For this review, use the dimensioned drawing (mm, ordinates from the lowest corner) and the shaded views. Coordinates: 2 decimals unless noted, no trailing zeros. Write each loop counter-clockwise with the first axis right and the second up, starting at its lowest first coordinate (ties: lowest second). Pieces come first, ordered by that corner, then holes. Notation, with made-up numbers: M 48,17.5 L 80,17.5 A15 ccw 80,25.5 Z; hole C -37.5,71 d4. An arc over 180 degrees is marked long. One line per question, with ' | ' between items.
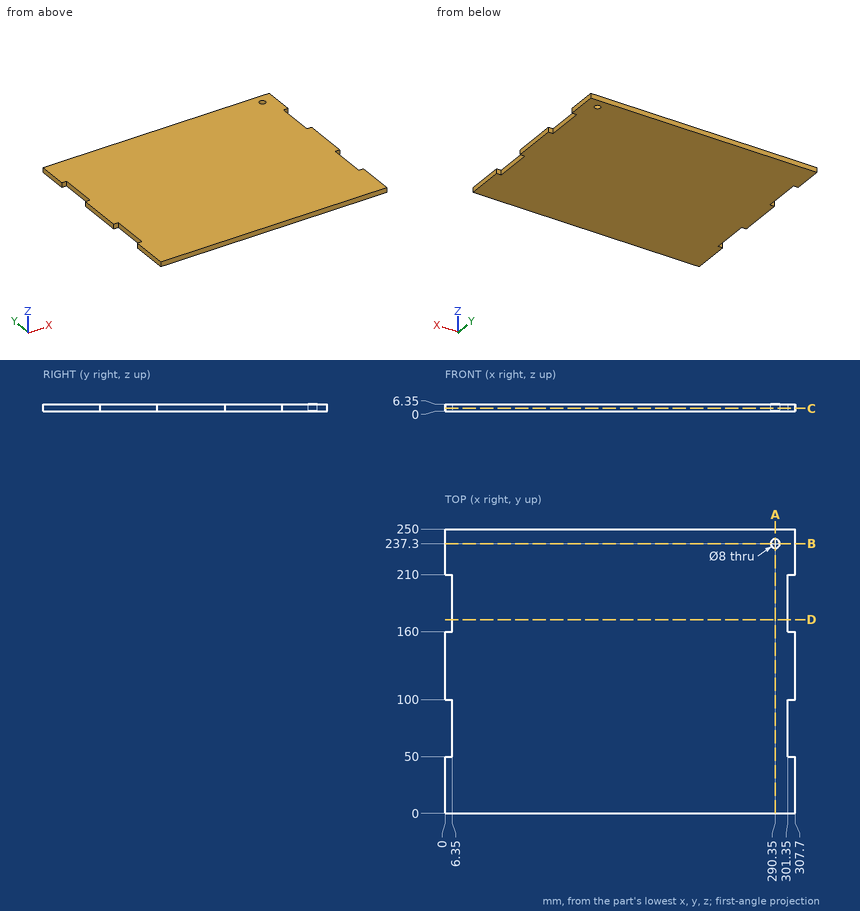
1) We need section C-C on z = 2.5. State the section outline as (x, y) points, then the cut area to 3 significant figures.
Responses:
outline: M 0,0 L 307.7,0 L 307.7,50 L 301.35,50 L 301.35,100 L 307.7,100 L 307.7,160 L 301.35,160 L 301.35,210 L 307.7,210 L 307.7,250 L 0,250 L 0,210 L 6.35,210 L 6.35,160 L 0,160 L 0,100 L 6.35,100 L 6.35,50 L 0,50 Z; hole C 290.35,237.3 d8 | area: 75,600 mm^2
2) Insertion check: pin 1 Ø3 at (y, z) = (65.5, 3) entering from +X; pin 2 Ø6.5 at (x, y) = (290.35, 237.3) entering from +Z; pin 3 Ø3 at (y, z) = (66, 2) entering from -X. Each pin has a flat end and moves straight along its axis. Give the tip position at first contact, or say it passes through.
Responses:
pin 1: x = 301.35 | pin 2: through | pin 3: x = 6.35
3) We need section D-D on y = 170.5. State the section outline as (x, z) points, then the cut area to 3 significant figures.
Responses:
outline: M 6.35,0 L 301.35,0 L 301.35,6.35 L 6.35,6.35 Z | area: 1,870 mm^2
4) We need section A-A on x = 290.35. State the section outline as (y, z) points.
Responses:
outline: M 0,0 L 233.3,0 L 233.3,6.35 L 0,6.35 Z; M 241.3,0 L 250,0 L 250,6.35 L 241.3,6.35 Z
5) We need section B-B on y = 237.3. State the section outline as (x, z) points, then the cut area to 3 significant figures.
Responses:
outline: M 0,0 L 286.35,0 L 286.35,6.35 L 0,6.35 Z; M 294.35,0 L 307.7,0 L 307.7,6.35 L 294.35,6.35 Z | area: 1,900 mm^2
6) To check wall thickness, follow line 1 along Y through (x, z) = (290.35, 4); line 2 along X through (y, z) = (55.5, 3.75). State the ranges of each line that lie inside material, in increasing order. Write a range as [from, to].
Responses:
line 1: [0, 233.3], [241.3, 250] | line 2: [6.35, 301.35]
